Here's the drawing with two shaded views (mm, measured from the low corner). I have some questions. Round coordinates to 2 decimals unless told otherwise and drop trailing zeros. Loops run counter-clockwise (first coordinate to the right, second up) from the corner with the lowest first, then second, coordinate; pieces in that order, holes last. Notation, with made-up numbers: M 82.5,-36 L 138.5,-36 A21 cw 138.5,-29 Z; hole C -0.5,63.25 d6. An arc over 180 degrees is marked long. Answer as a JSON object with one key per item and string values.
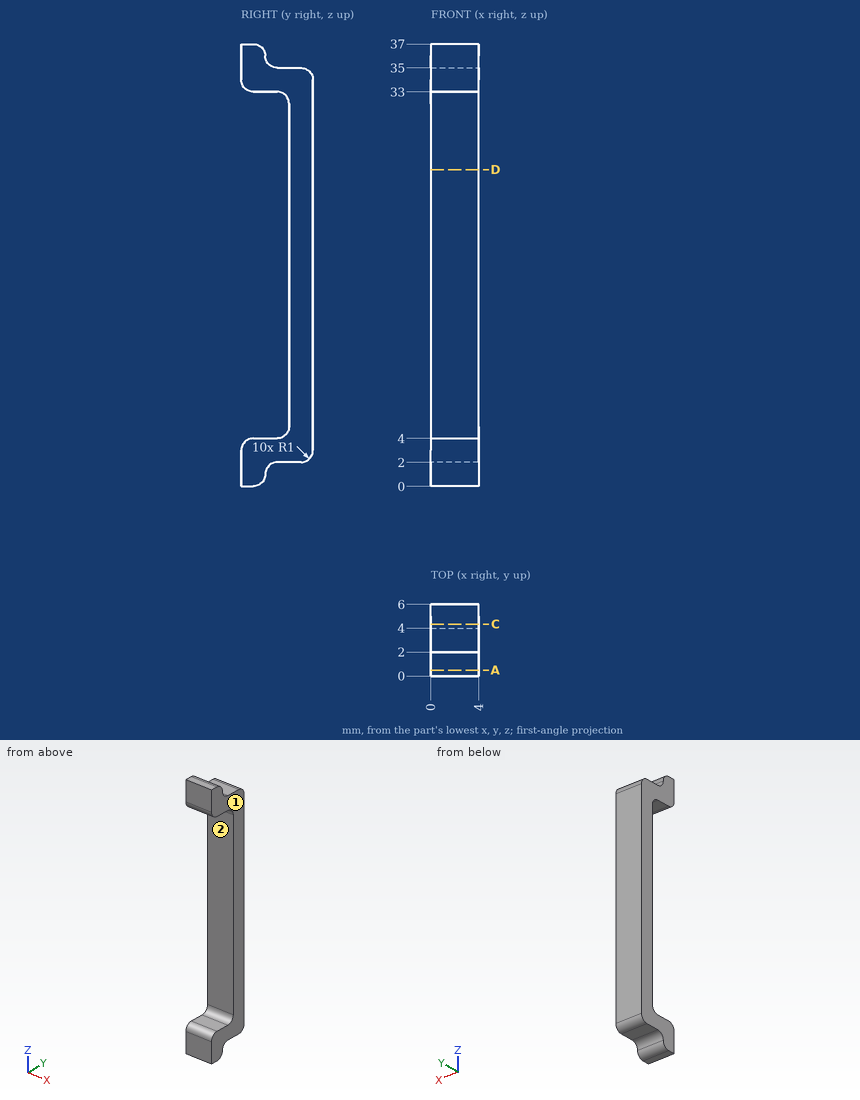
Item 1: I want a section at A-A on y = 0.5. List the corners of the cut face in (x, z) for me.
Solution:
{"outline": "M 0,0 L 4,0 L 4,3.87 L 0,3.87 Z; M 0,33.13 L 4,33.13 L 4,37 L 0,37 Z"}
Item 2: If I drill on L1, parallel to Z at x = 0.85, y = 4.55; L2, parallel to Y at x = 3.35, z = 5; L3, parallel to Y at x = 2.9, z = 36, over which ranges is the centre line in solid material (lowest first)? Write a range as from..to.
Solution:
{"L1": "z = 2..35", "L2": "y = 4..6", "L3": "y = 0..2"}
Item 3: I want a section at D-D on z = 26.5. List the corners of the cut face in (x, y) for me.
Solution:
{"outline": "M 0,4 L 4,4 L 4,6 L 0,6 Z"}
Item 4: For P1, Ø1.6, axis at x = 1, y = 2, coming from the +Z side; P2, Ø0.6, axis at x = 1.5, y = 4, coming from the -Z side; P3, Ø1.6, axis at x = 1, y = 3.5, coming from the +Z side (1 decimal), each with a flat end and sliding along its axis, tell me the tip position at first contact or that it passes through.
Solution:
{"P1": "stops at z = 36.98", "P2": "stops at z = 2", "P3": "stops at z = 35"}
Item 5: We'd pull the mould along Z, two halves only. Please class the marked faces 1 and 2: +Z half, -Z half, draft (parallel to the pull), parting line (faces both ways), or undercut.
Solution:
{"face 1": "draft", "face 2": "undercut"}
Item 6: I want a section at C-C on y = 4.35. List the corners of the cut face in (x, z) for me.
Solution:
{"outline": "M 0,2 L 4,2 L 4,35 L 0,35 Z"}
